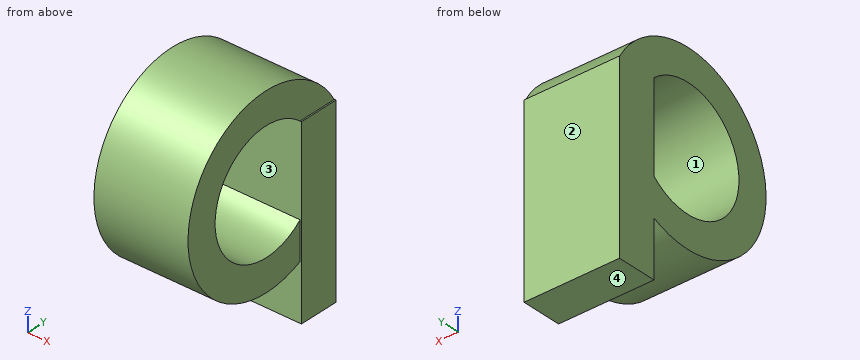
from build123d import *

# Parameters (mm, degrees)
F0_R     = 24.6246836301
F1_DEPTH = 25.4
F2_R     = 16.0828148766
F3_DEPTH = 25.401
F4_W     = 28.0453877614
F4_H     = 49.2377767596
F5_DEPTH = 25.77823
F6_DEPTH = 17.15412


with BuildPart() as f1:
    # F0 (on Right) → F1 (new body)
    with BuildSketch(Plane.YZ):
        with Locations((0, 37.2249111533)):
            Circle(F0_R)
    extrude(amount=-F1_DEPTH)

    # F2 (on face) → F3 (cut, through all)
    with BuildSketch(Plane(origin=(-25.4, 0, 0), x_dir=(0, -1, 0), z_dir=(-1, 0, 0))):
        with Locations((0, 37.2249111533)):
            Circle(F2_R)
    extrude(amount=-F3_DEPTH, mode=Mode.SUBTRACT)

    # F4 (on face) → F5 (join)
    with BuildSketch(Plane(origin=(-25.4, 0, 0), x_dir=(0, -1, 0), z_dir=(-1, 0, 0))):
        with Locations((-24.7160560406, 24.6188883798)):
            Rectangle(F4_W, F4_H)
    extrude(amount=-F5_DEPTH)

    # F6 (cut): a face of the model
    f6_faces = [f1.faces().sort_by_distance(p)[0] for p in [
        (-12.510885, 38.7387499213, 24.6188883798),
    ]]
    extrude(f6_faces, amount=-F6_DEPTH, mode=Mode.SUBTRACT)


solid = f1.part
Model file for the job. Use its own axes, mm. Face numbers are marked on the shaded views. Round coordinates to 2 decimals unless told otherwise and drop trailing zeros. Order: outer loops, then holes, each group sorted by start corner. A loop starts at its lowest first (then second) coordinate and runs counter-clockwise, first axis right, second up.
(1) Band-saw the part on C-C (x = -4.5). List the corners of the cut face in (y, z), then the cut area to 3 significant figures.
(2) Drill centre lines: line 1 (Z direction, x = -7, y = 0); line 2 (Y direction, x = -8.75, z = 37); line 3 (Y direction, x = -3, z = 51.5). Where is each one in solid material? Low to high.
(3) Band-saw the part on A-A (y = 0). List the corners of the cut face in (x, z), then the cut area to 3 significant figures.
(4) Pin check, flat tips, straight feed: pin 1 (23 mm diameter, centred on y = -1.5, z = 28, fed in from +X); pin 2 (5.5 mm diameter, centred on x = -17, y = 15, fed in from +Z); pin 3 (1 mm diameter, centred on x = -11.5, y = -10.5, fed in from -Z). Stop position of each tip, or through.
(5) Band-saw the part on B-B (z = 45). List the corners of the cut face in (x, y) (3 decimals), then the cut area to 3 significant figures.
(6) Pull direction Y, two halves, no side cores. Call the marked faces 1, 2, 3 and 4: released by +Y, released by -Y, zero draft, split by the parting line, or undercut.
Verdict:
1. outline: (10.69, 0) - (21.58, 0) - (21.58, 49.24) - (21.5, 49.24) arc R24.62 ccw (long way) to (10.69, 15.04) - close; hole (10.69, 25.21) - (10.69, 49.24) arc R16.08 ccw (long way) to start
1. area: 1,340 mm2
2. line 1: z = 12.6 to 21.14, 53.31 to 61.85
2. line 2: y = -24.62 to -16.08, 10.69 to 21.58
2. line 3: y = -20.06 to -7.41, 7.41 to 20.06
3. outline: (-25.4, 12.6) - (0, 12.6) - (0, 21.14) - (-25.4, 21.14) - close; (-25.4, 53.31) - (0, 53.31) - (0, 61.85) - (-25.4, 61.85) - close
3. area: 434 mm2
4. pin 1: stops at x = 0
4. pin 2: stops at z = 58.59
4. pin 3: stops at z = 14.72
5. outline: (-25.4, -23.365) - (0, -23.365) - (0, -14.079) - (-25.4, -14.079) - close; (-25.4, 10.693) - (0.378, 10.693) - (0.378, 21.585) - (-25.4, 21.585) - close
5. area: 517 mm2
6. face 1: undercut
6. face 2: released by +Y
6. face 3: undercut
6. face 4: zero draft
